Part model, mm, in its own coordinate system. A direction names the side the tool comes from. Give positions to 0.01 mm unless a question says otherwise; leave off trailing zeros. Order: outer loops, then holes, each group sorted by start corner. A loop starts at its lowest first (then second) coordinate and runs counter-clockwise, first axis right, second up. Notation, with made-up numbers: (32, 32) -> (38, 32) arc R11 cw to (38, 48) -> close; hole circle Ø1 at (47.25, 43). An arc over 180 degrees is marked (long way). Write item = value, one per line. Start each with the question number.
Item 1: Drill centre lines: line 1 along Y through (x, z) = (-0.5, 3.5); line 2 along Y through (x, z) = (-30.5, 5); line 3 along X through (y, z) = (10.5, 5.5). Where is each one in solid material? Low to high.
Item 2: Pull direction Y, two halves, no side cores. Call faces 6 (the face through (7.74, 56.33, 1.25)), 7 (the face through (-33.42, 29.33, 1.25)), 8 (the face through (-10.68, -10.44, 5.1)): +Y half, -Y half, draft (parallel to the pull), parting line (faces both ways), or undercut.
Item 3: Band-saw the part on A-A on y = 54.5. Write the cut outline in (x, z), plus the area to 3 significant figures.
Item 4: Band-saw the part on D-D on x = 12. Count the separate pieces of the cut face and the enclosed holes in it, plus the area to 3 significant figures.
Item 5: Flat gauge pins, fed straight in: P1, Ø1.4, axis at y = -15.5, z = 3, coming from the +X side; P2, Ø1.4, axis at x = -12.5, z = 3.5, coming from the -Y side. Where does each tip first touch, or does it go through?
Item 6: Band-saw the part on C-C on y = -1.5. Write the cut outline in (x, z).
Item 7: Tool access for faces 1 (the face through (-28.88, -24.32, 1.25)), 2 (the face through (13.397, 2.041, 3.166)), 3 (the face through (1.7, 46.36, 2.1)), 4 (the face through (-36.34, -19.71, 1.25)), 5 (the face through (1.636, -14.162, 4.251)): list every direction of +Z, -Z, +X, -X, +Y, -Y with a clear straight run to the whole face (end or side of a thin tool).
```python
from build123d import *

# Parameters (mm, degrees)
F0_R     = 11
F1_DEPTH = 6.35
F2_SIZE  = 2.54


with BuildPart() as f1:
    # F0 (on Top) → F1 (new body)
    with BuildSketch(Plane.XY):
        with BuildLine():
            ThreePointArc((-45.635105, 5.008696), (-44.147658, 10.559926), (-38.596428, 9.072478))
            Line((-38.596428, 9.072478), (-30.58888, -4.797003))
            ThreePointArc((-30.58888, -4.797003), (-32.076327, -10.348232), (-37.627557, -8.860785))
            Line((-37.627557, -8.860785), (-37.627557, -30.85783))
            Line((-37.627557, -30.85783), (-18.577557, -19.859307))
            ThreePointArc((-18.577557, -19.859307), (-22.641339, -15.795525), (-18.577557, -11.731743))
            Line((-18.577557, -11.731743), (-2.562459, -11.731743))
            ThreePointArc((-2.562459, -11.731743), (1.501323, -15.795525), (-2.562459, -19.859307))
            Line((-2.562459, -19.859307), (16.487541, -30.85783))
            Line((16.487541, -30.85783), (16.487541, -8.860785))
            ThreePointArc((16.487541, -8.860785), (10.936311, -10.348232), (9.448863, -4.797003))
            Line((9.448863, -4.797003), (17.456412, 9.072478))
            ThreePointArc((17.456412, 9.072478), (23.007642, 10.559926), (24.495089, 5.008696))
            Line((24.495089, 5.008696), (43.545089, 16.007219))
            Line((43.545089, 16.007219), (24.495089, 27.005742))
            ThreePointArc((24.495089, 27.005742), (23.007642, 21.454512), (17.456412, 22.941959))
            Line((17.456412, 22.941959), (9.448863, 36.81144))
            ThreePointArc((9.448863, 36.81144), (10.936311, 42.36267), (16.487541, 40.875223))
            Line((16.487541, 40.875223), (16.487541, 62.872268))
            Line((16.487541, 62.872268), (-2.562459, 51.873745))
            ThreePointArc((-2.562459, 51.873745), (1.501323, 47.809963), (-2.562459, 43.746181))
            Line((-2.562459, 43.746181), (-18.577557, 43.746181))
            ThreePointArc((-18.577557, 43.746181), (-22.641339, 47.809963), (-18.577557, 51.873745))
            Line((-18.577557, 51.873745), (-37.627557, 62.872268))
            Line((-37.627557, 62.872268), (-37.627557, 40.875223))
            ThreePointArc((-37.627557, 40.875223), (-32.076327, 42.36267), (-30.58888, 36.81144))
            Line((-30.58888, 36.81144), (-38.596428, 22.941959))
            ThreePointArc((-38.596428, 22.941959), (-44.147658, 21.454512), (-45.635105, 27.005742))
            Line((-45.635105, 27.005742), (-64.685105, 16.007219))
            Line((-64.685105, 16.007219), (-45.635105, 5.008696))
        make_face()
        with Locations((-10.570008, 16.007219)):
            Circle(F0_R, mode=Mode.SUBTRACT)
    extrude(amount=F1_DEPTH)

    # F2
    f2_edges = [f1.edges().sort_by_distance(p)[0] for p in [
        (-44.147658, 21.454512, 6.35),
        (-55.160105, 21.50648, 6.35),
        (-55.160105, 10.507958, 6.35),
        (-44.147658, 10.559926, 6.35),
        (-34.592654, 2.137738, 6.35),
        (-32.076327, -10.348232, 6.35),
        (-37.627557, -19.859307, 6.35),
        (-28.102557, -25.358569, 6.35),
        (-22.641339, -15.795525, 6.35),
        (-10.570008, -11.731743, 6.35),
        (1.501323, -15.795525, 6.35),
        (6.962541, -25.358569, 6.35),
        (16.487541, -19.859307, 6.35),
        (10.936311, -10.348232, 6.35),
        (13.452638, 2.137738, 6.35),
        (23.007642, 10.559926, 6.35),
        (34.020089, 10.507958, 6.35),
        (34.020089, 21.50648, 6.35),
        (23.007642, 21.454512, 6.35),
        (13.452638, 29.8767, 6.35),
        (10.936311, 42.36267, 6.35),
        (16.487541, 51.873745, 6.35),
        (6.962541, 57.373007, 6.35),
        (1.501323, 47.809963, 6.35),
        (-10.570008, 43.746181, 6.35),
        (-22.641339, 47.809963, 6.35),
        (-28.102557, 57.373007, 6.35),
        (-37.627557, 51.873745, 6.35),
        (-32.076327, 42.36267, 6.35),
        (-34.592654, 29.8767, 6.35),
        (-21.570008, 16.007219, 6.35),
        (-44.147658, 21.454512, 0),
        (-55.160105, 21.50648, 0),
        (-55.160105, 10.507958, 0),
        (-44.147658, 10.559926, 0),
        (-34.592654, 2.137738, 0),
        (-32.076327, -10.348232, 0),
        (-37.627557, -19.859307, 0),
        (-28.102557, -25.358569, 0),
        (-22.641339, -15.795525, 0),
        (-10.570008, -11.731743, 0),
        (1.501323, -15.795525, 0),
        (6.962541, -25.358569, 0),
        (16.487541, -19.859307, 0),
        (10.936311, -10.348232, 0),
        (13.452638, 2.137738, 0),
        (23.007642, 10.559926, 0),
        (34.020089, 10.507958, 0),
        (34.020089, 21.50648, 0),
        (23.007642, 21.454512, 0),
        (13.452638, 29.8767, 0),
        (10.936311, 42.36267, 0),
        (16.487541, 51.873745, 0),
        (6.962541, 57.373007, 0),
        (1.501323, 47.809963, 0),
        (-10.570008, 43.746181, 0),
        (-22.641339, 47.809963, 0),
        (-28.102557, 57.373007, 0),
        (-37.627557, 51.873745, 0),
        (-32.076327, 42.36267, 0),
        (-34.592654, 29.8767, 0),
        (-21.570008, 16.007219, 0),
    ]]
    chamfer(f2_edges, length=F2_SIZE)


solid = f1.part
```
Values found:
q1.line_1 = -21.05 to -19.3, -12.29 to 11.58, 20.43 to 44.31, 51.31 to 53.06
q1.line_2 = -25.37 to -10.65, -2.57 to 34.59, 42.66 to 57.38
q1.line_3 = -51.77 to -46.71, -37.52 to -22, 0.86 to 16.38, 25.57 to 30.63
q2.face_6 = +Y half
q2.face_7 = undercut
q2.face_8 = -Y half
q3.outline = (-37.63, 2.54) -> (-35.09, 0) -> (-28.21, 0) -> (-23.13, 2.54) -> (-23.13, 3.81) -> (-28.21, 6.35) -> (-35.09, 6.35) -> (-37.63, 3.81) -> close; (1.99, 2.54) -> (7.07, 0) -> (13.95, 0) -> (16.49, 2.54) -> (16.49, 3.81) -> (13.95, 6.35) -> (7.07, 6.35) -> (1.99, 3.81) -> close
q3.area = 145 mm^2
q4.separate_pieces = 3
q4.enclosed_holes = 0
q4.area = 376 mm^2
q5.P1 = 16.49
q5.P2 = -11.73
q6.outline = (-32.49, 2.54) -> (-29.56, 0) -> (8.42, 0) -> (11.35, 2.54) -> (11.35, 3.81) -> (8.42, 6.35) -> (-29.56, 6.35) -> (-32.49, 3.81) -> close
q7.face_1 = -Z, -Y
q7.face_2 = +Z, -Z
q7.face_3 = -Z
q7.face_4 = -Z, -X, -Y
q7.face_5 = +Z
